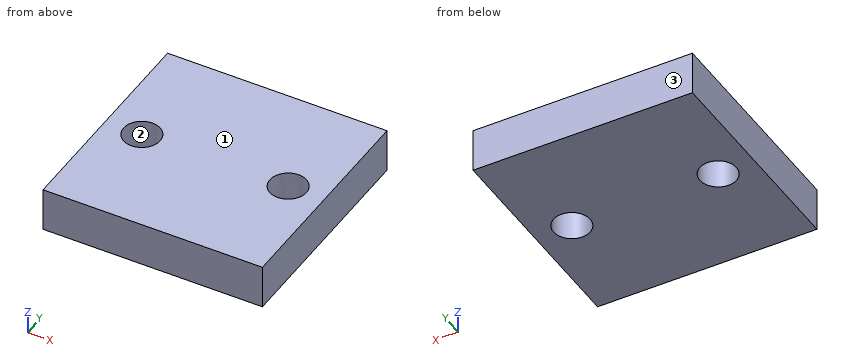
Autodesk Inventor part; units mm, degrees
ref_plane "YZ Plane" through (0, 0, 0) normal (1, 0, 0) x (0, 1, 0)
ref_plane "XZ Plane" through (0, 0, 0) normal (0, 1, 0) x (-1, 0, 0)
ref_plane "XY Plane" through (0, 0, 0) normal (0, 0, 1) x (1, 0, 0)
sketch "Sketch1" plane through (0, 0, 0) normal (0, 0, 1) x (1, 0, 0)
  point P0 (0, 0)
sketch "Sketch2" plane through (0, 0, 0) normal (0, 0, 1) x (1, 0, 0)
  line L0 (0, 0) -> (30, 0)
  line L1 (30, 0) -> (30, 30)
  line L2 (30, 30) -> (0, 30)
  line L3 (0, 30) -> (0, 0)
  dimension "d0" = 30
  dimension "d1" = 30
extrude "Extrusion1" add sketch "Sketch2" along normal blind 6
sketch "Sketch3" plane through (0, 0, 6) normal (0, 0, 1) x (1, 0, 0)
  circle A0 centre (5, 15) radius 2.5
  circle A1 centre (25, 15) radius 2.5
  line L0 (0, 0) -> (30, 0)
  line L1 (30, 0) -> (30, 30)
  line L2 (0, 30) -> (0, 0)
  dimension "d4" = 15
  dimension "d5" = 15
  dimension "d6" = 5
  dimension "d7" = 5
  dimension "d8" = 5
extrude "Extrusion2" cut sketch "Sketch3" against normal blind 6
properties part number "space_plate"
CAD build for the part. Positions are in the model's coordinates, mm. Face numbers are marked on the shaded views. Round coordinates to 2 decimals unless told otherwise and drop trailing zeros. Write each loop counter-clockwise with the first axis right and the second up, starting at its lowest first coordinate (ties: lowest second). Pieces come first, ordered by that corner, then holes. Notation, with made-up numbers: (84.5, -36.75) -> (131.5, -36.75) arc R23 ccw to (131.5, -0.75) -> close; hole circle Ø7 at (46, 9). An arc over 180 degrees is marked (long way). Answer as a JSON object with one key per item and string values.
(1) Two-plate mould, pull along Y, no slides. Class the marked faces 1, 2 and 3: +Y half, -Y half, draft (parallel to the pull), parting line (faces both ways), or undercut.
Reported:
{"face 1": "draft", "face 2": "undercut", "face 3": "+Y half"}
(2) Band-saw the part on D-D, the plane x = 23.5. List the corners of the cut face in (y, z), then the cut area to 3 significant figures.
Reported:
{"outline": "(0, 0) -> (13, 0) -> (13, 6) -> (0, 6) -> close; (17, 0) -> (30, 0) -> (30, 6) -> (17, 6) -> close", "area": "156 mm^2"}
(3) Pin check, flat tips, straight feed: P1, Ø3, axis at x = 5, y = 15, coming from the -Z side; P2, Ø5, axis at x = 11, y = 6, coming from the -Z side. Stop position of each tip, or through.
Reported:
{"P1": "passes through", "P2": "stops at z = 0"}
(4) Probe probe 1 along Y at (x, z) = (25, 1.85); probe 2 along X at (y, z) = (15.5, 1.2); probe 3 along X at (y, z) = (17, 5.3). List the from-to ranges inside material, lowest first. Write a range as [from, to].
Reported:
{"probe 1": "y = [0, 12.5], [17.5, 30]", "probe 2": "x = [0, 2.55], [7.45, 22.55], [27.45, 30]", "probe 3": "x = [0, 3.5], [6.5, 23.5], [26.5, 30]"}
(5) Band-saw the part on A-A, the plane x = 5. List the corners of the cut face in (y, z).
Reported:
{"outline": "(0, 0) -> (12.5, 0) -> (12.5, 6) -> (0, 6) -> close; (17.5, 0) -> (30, 0) -> (30, 6) -> (17.5, 6) -> close"}
(6) Band-saw the part on B-B, the plane y = 15. List the corners of the cut face in (x, z).
Reported:
{"outline": "(0, 0) -> (2.5, 0) -> (2.5, 6) -> (0, 6) -> close; (7.5, 0) -> (22.5, 0) -> (22.5, 6) -> (7.5, 6) -> close; (27.5, 0) -> (30, 0) -> (30, 6) -> (27.5, 6) -> close"}
(7) Band-saw the part on C-C, the plane z = 3.1. List the corners of the cut face in (x, y), then the cut area to 3 significant figures.
Reported:
{"outline": "(0, 0) -> (30, 0) -> (30, 30) -> (0, 30) -> close; hole circle Ø5 at (5, 15); hole circle Ø5 at (25, 15)", "area": "861 mm^2"}
